from build123d import *

# Parameters (mm, degrees)
F1_DEPTH = 554
F2_R     = 2


with BuildPart() as f1:
    # F0 (on Right) → F1 (new body)
    with BuildSketch(Plane.YZ):
        Polygon((-21, 40), (-40, 40), (-40, 18), (-34, 18), (-34, 21), (-28, 21), (-28, 9), (-34, 9), (-34, 12), (-40, 12), (-40, -12), (-34, -12), (-34, -9), (-28, -9), (-28, -21), (-34, -21), (-34, -18), (-40, -18), (-40, -40), (-18, -40), (-18, -34), (-21, -34), (-21, -28), (-9, -28), (-9, -34), (-12, -34), (-12, -40), (15, -40), (15, -34), (12, -34), (12, -28), (24, -28), (24, -34), (21, -34), (21, -40), (40, -40), (40, -18), (34, -18), (34, -21), (28, -21), (28, -9), (34, -9), (34, -12), (40, -12), (40, 12), (34, 12), (34, 9), (28, 9), (28, 21), (34, 21), (34, 18), (40, 18), (40, 40), (21, 40), (21, 34), (24, 34), (24, 28), (12, 28), (12, 34), (15, 34), (15, 40), (-15, 40), (-15, 34), (-12, 34), (-12, 28), (-24, 28), (-24, 34), (-21, 34), align=None)
    extrude(amount=F1_DEPTH)

    # F2
    f2_edges = [f1.edges().sort_by_distance(p)[0] for p in [
        (277, 40, 40),
        (277, 40, -40),
        (277, -40, 40),
        (277, -40, -40),
        (277, -40, -18),
        (277, -40, -12),
        (277, -40, 12),
        (277, -40, 18),
        (277, 21, 40),
        (277, 15, 40),
        (277, -15, 40),
        (277, -21, 40),
        (277, 40, 18),
        (277, 40, 12),
        (277, 40, -12),
        (277, 40, -18),
        (277, 21, -40),
        (277, 15, -40),
        (277, -12, -40),
        (277, -18, -40),
    ]]
    fillet(f2_edges, radius=F2_R)


solid = f1.part
Work out the finished part from the listing and answer in its coordinate system (mm). A direction names the side the tool comes from. Give positions to 0.01 mm unless a question says otherwise; leave off trailing zeros. Return JSON: item names as keys, results as strings.
Q1. Which of the six approach directions +Z, -Z, +X, -X, +Y, -Y give full straight-line access (tool end or side, diameter ignored) to faces 5 (the face through (273, -28, 15)), 6 (the face through (273, 31, 40))?
Answer below:
{"face 5": "+X, -X", "face 6": "+Z, +X, -X, +Y, -Y"}
Q2. Find the intervals of material crossed by line 1 along Y through (x, z) = (302, 36.5); line 2 along Z through (x, y) = (163.5, -35.5); line 3 along Y through (x, z) = (261, -31), in increasing order. Write a range as [from, to].
Answer below:
{"line 1": "y = [-40, -21], [-15, 15], [21, 40]", "line 2": "z = [-40, -18], [-12, 12], [18, 40]", "line 3": "y = [-40, -21], [-9, 12], [24, 40]"}
Q3. The mould has two halves that part along Y. Classify faces 1 (the face through (273, -28, -15)), 2 (the face through (273, -30, 40)), 3 (the face through (273, -40, -29)), 4 (the face through (273, -15, -28)): pulls with the +Y half, pulls with the -Y half, needs draft (parallel to the pull), parting line crosses it, or undercut.
Answer below:
{"face 1": "undercut", "face 2": "needs draft", "face 3": "pulls with the -Y half", "face 4": "undercut"}
Q4. Each of these flat-tipped pins is pushed along its axis until it touches: pin 1 (0.9 mm diameter, centred on x = 165, z = -11, fed in from -Y); pin 2 (2.5 mm diameter, centred on x = 408, y = -20, fed in from +Z); pin 3 (4 mm diameter, centred on x = 112, y = 16.5, fed in from -Z). Where does it stop, or does it pass through?
Answer below:
{"pin 1": "stops at y = -39.92", "pin 2": "stops at z = 38.97", "pin 3": "stops at z = -39.32"}
